Autodesk Inventor part; units mm, degrees
ref_plane "YZ Plane" through (0, 0, 0) normal (1, 0, 0) x (0, 1, 0)
ref_plane "XZ Plane" through (0, 0, 0) normal (0, 1, 0) x (-1, 0, 0)
ref_plane "XY Plane" through (0, 0, 0) normal (0, 0, 1) x (1, 0, 0)
sketch "Sketch1" plane through (0, 0, 0) normal (0, 1, 0) x (-1, 0, 0)
  line L0 (0, 0) -> (3.5, 0)
  line L1 (3.5, 0) -> (3.5, -1.5)
  line L2 (3.5, -1.5) -> (2, -1.5)
  line L3 (2, -1.5) -> (2, -4)
  line L4 (2, -4) -> (3, -4)
  line L5 (3, -4) -> (1.5, -6.5981)
  line L6 (1.5, -6.5981) -> (0, -6.5981)
  line L7 (0, -6.5981) -> (0, 0)
  line L8 (0, -7.9177) -> (0, 1.3196)
  dimension "d0" = 3.5
  dimension "d1" = 1.5
  dimension "d3" = 2.5
  dimension "d4" = 2
  dimension "d5" = 1
  dimension "d6" = 1.5
  dimension "d7" = 60
revolve "Revolution1" add sketch "Sketch1" angle 360 about axis through (0, 0, -10) along (0, 0, 1)
sketch "Sketch2" plane through (0, 0, 0) normal (0, 0, 1) x (1, 0, 0)
  circle A0 centre (0, 0) radius 3.5 construction
  line L0 (-1.5, 0) -> (1.5, 0)
  line L1 (1.5, 0) -> (1.5, 18)
  line L2 (1.5, 18) -> (-1.5, 18)
  line L3 (-1.5, 18) -> (-1.5, 0)
  line L4 (-5.5, 18) -> (5.5, 18)
  line L5 (5.5, 18) -> (5.5, 35)
  line L6 (5.5, 35) -> (-5.5, 35)
  line L7 (-5.5, 35) -> (-5.5, 18)
  point P0 (0, 18)
  dimension "d9" = 3
  dimension "d10" = 18
  dimension "d11" = 11
  dimension "d12" = 17
extrude "Extrusion1" add sketch "Sketch2" against normal blind 1
sketch "Sketch3" plane through (0, 0, -1) normal (0, 0, -1) x (-1, 0, 0)
  line L0 (3.5, 33) -> (-3.5, 33)
  line L1 (-3.5, 33) -> (-3.5, 20)
  line L2 (-3.5, 20) -> (3.5, 20)
  line L3 (3.5, 20) -> (3.5, 33)
  line L4 (5.5, 35) -> (-5.5, 35)
  line L5 (5.5, 18) -> (5.5, 35)
  point P0 (0, 0)
  point P1 (0, 33)
  point P2 (0, 35)
  point P3 (3.5, 26.5)
  point P4 (5.5, 26.5)
  dimension "d15" = 7
  dimension "d16" = 13
extrude "Extrusion2" add sketch "Sketch3" along normal blind 3
sketch "Sketch4" plane through (0, 0, -4) normal (0, 0, -1) x (-1, 0, 0)
  line L0 (-3.5, 33) -> (-3.5, 20)
  line L1 (-3.5, 20) -> (3.5, 20)
  line L2 (3.5, 20) -> (3.5, 33)
  line L3 (3.5, 33) -> (-3.5, 33)
  line L4 (4.2, 33.7) -> (4.2, 19.3)
  line L5 (4.2, 19.3) -> (-4.2, 19.3)
  line L6 (-4.2, 19.3) -> (-4.2, 33.7)
  line L7 (-4.2, 33.7) -> (4.2, 33.7)
  point P0 (0, 0)
  dimension "d20" = 0.7
extrude "Extrusion3" add sketch "Sketch4" along normal blind 1 contours L3 L2 L1 L0 | L4 L5 L6 L7
fillet "Fillet1" radius 2 12 edges at (-5.5, 35, -0.5) (-5.5, 18, -0.5) (5.5, 35, -0.5) (5.5, 18, -0.5) (3.5, 20, -2.5) (3.5, 33, -2.5) (-3.5, 33, -2.5) (-3.5, 20, -2.5) (-4.2, 19.3, -4.5) (4.2, 19.3, -4.5) (4.2, 33.7, -4.5) (-4.2, 33.7, -4.5)
chamfer "Chamfer1" distance 0.5 angle 45 8 edges at (-4.2, 26.5, -5) (-3.6142, 33.1142, -5) (0, 33.7, -5) (3.6142, 33.1142, -5) (4.2, 26.5, -5) (3.6142, 19.8858, -5) (0, 19.3, -5) (-3.6142, 19.8858, -5)
fillet "Fillet2" radius 2 3 edges at (1.5, 3.1623, -0.5) (0, 3.5, -1) (-1.5, 3.1623, -0.5)
properties part number "USB-C_cover" material "PC/ABS Plastic"
Design review of the part built by this model. Coordinates are the model's own, in mm. A direction names the side the tool comes from. Give positions to 0.01 mm unless a question says otherwise; leave off trailing zeros. Loops run counter-clockwise (first coordinate to the right, second up) from the corner with the lowest first, then second, coordinate; pieces in that order, holes last. Notation, with made-up numbers: M 39,40.25 L 51,40.25 A5 ccw 51,46.25 Z; hole C 64,-3.75 d7. An arc over 180 degrees is marked long. Return JSON: item names as keys, results as strings. Group by question number.
Item 1: For probe 1 along Z at (x, y) = (-3.5, 31.5); probe 2 along Z at (x, y) = (2.25, 27); probe 3 along Y at (x, z) = (-1.5, -3.75), list the stretches that pass through material, from the lowest coordinate up.
Item 2: We need section A-A (z = -2.5). Give the boundary of the cut face in (x, y).
Item 3: We need section B-B (y = 28.5). Give the boundary of the cut face in (x, z), and give its area (4 significant figures).
Item 4: Tool access review of faces 5 (the flat face through (-1, 2, -4)), 6 (the flat face through (1.5, 11, -0.5)), 7 (the flat face through (-3.5, 26, -2)): name each direction out of +Z, -Z, +X, -X, +Y, -Y from which nothing blocks a thin tool from reaching the whole face with its end or side.
Item 5: We need section C-C (x = 0). Give the boundary of the cut face in (y, z), and give its area (3 significant figures).
Item 6: Mouldability with a two-part tool opening along Z and no side actions: class faces 1 (the flat face through (2.4, 20, -1)), 2 (the cylindrical face through (-2.9, 20.57, -2.52)), 3 (the flat face through (2.5, 18, -0.5)), 4 (the flat face through (0, 20, 0)) as released by +Z, released by -Z, zero draft, split by the parting line, or undercut.
Item 7: Insertion check: pin 1 Ø3 at (x, y) = (-4, 21) entering from +Z; pin 2 Ø0.6 at (y, z) = (25, -4) entering from -X; pin 3 Ø2.5 at (x, z) = (-0.5, -3) entering from -Y; pin 4 Ø3.5 at (x, y) = (-0.5, 24.5) entering from -Z. Each pin has a flat end and moves straight along its axis. Give the tip position at first contact, or say it passes through.
Item 8: We need section D-D (y = 0). Give the boundary of the cut face in (x, z), and give its area (3 significant figures).
Output:
{
 "1": {"probe 1": "z = -5 to -4, -1 to 0", "probe 2": "z = -5 to 0", "probe 3": "y = -1.32 to 1.32, 20 to 33"},
 "2": {"outline": "M -3.5,22 A2 ccw -1.5,20 L 1.5,20 A2 ccw 3.5,22 L 3.5,31 A2 ccw 1.5,33 L -1.5,33 A2 ccw -3.5,31 Z; C 0,0 d4"},
 "3": {"outline": "M -5.5,-1 L -3.5,-1 L -3.5,-4 L -4.2,-4 L -4.2,-4.5 L -3.7,-5 L 3.7,-5 L 4.2,-4.5 L 4.2,-4 L 3.5,-4 L 3.5,-1 L 5.5,-1 L 5.5,0 L -5.5,0 Z", "area": "40.15 mm^2"},
 "4": {"face 5": "none", "face 6": "+Z, -Z, +X", "face 7": "-X, +Y, -Y"},
 "5": {"outline": "M -3.5,-1.5 L -2,-1.5 L -2,-4 L -3,-4 L -1.5,-6.6 L 1.5,-6.6 L 3,-4 L 2,-4 L 2,-1.5 L 3.5,-1.5 A2 cw 4.82,-1 L 20,-1 L 20,-4 L 19.3,-4 L 19.3,-4.5 L 19.8,-5 L 33.2,-5 L 33.7,-4.5 L 33.7,-4 L 33,-4 L 33,-1 L 35,-1 L 35,0 L -3.5,0 Z", "area": "117 mm^2"},
 "6": {"face 1": "undercut", "face 2": "undercut", "face 3": "zero draft", "face 4": "released by +Z"},
 "7": {"pin 1": "stops at z = 0", "pin 2": "stops at x = -4.2", "pin 3": "stops at y = -3", "pin 4": "stops at z = -5"},
 "8": {"outline": "M -3.5,-1.5 L -2,-1.5 L -2,-4 L -3,-4 L -1.5,-6.6 L 1.5,-6.6 L 3,-4 L 2,-4 L 2,-1.5 L 3.5,-1.5 L 3.5,0 L -3.5,0 Z", "area": "32.2 mm^2"}
}
